```python
from build123d import *

# Parameters (mm, degrees)
EXTRUDE_1_DEPTH     = 2.5
FILLET_1_R          = 5
FILLET_2_R          = 10
FILLET_3_R          = 5
FILLET_4_R          = 1
EXTRUDE_2_DEPTH     = 12
SKETCH_3_R          = 2
CUT_EXTRUDE_1_DEPTH = 128.145329142
SHELL_1_T           = -1.2
CUT_EXTRUDE_2_DEPTH = 127.419500089
SKETCH_5_W          = 29.908945793
SKETCH_5_H          = 26
CUT_EXTRUDE_3_DEPTH = 12
CUT_EXTRUDE_4_DEPTH = 25
SKETCH_7_W          = 24.826968957
SKETCH_7_H          = 53.255380941
CUT_EXTRUDE_5_DEPTH = 140


with BuildPart() as part:
    # 草图1 → 凸台-拉伸1 (new body)
    with BuildSketch(Plane.XY):
        with BuildLine():
            Line((17, 0), (17, 14))
            Line((17, 14), (0, 14))
            Line((0, 14), (0, 43))
            Line((0, 43), (50, 43))
            Line((50, 43), (55, 46))
            Line((55, 46), (117, 46))
            Line((117, 46), (117, 43))
            Line((117, 43), (117, 0))
            ThreePointArc((117, 0), (93.5, -2.800462964), (70, 0))
            Line((70, 0), (17, 0))
        make_face()
    extrude(amount=EXTRUDE_1_DEPTH)

    # 圆角1
    fillet_1_edges = [part.edges().sort_by_distance(p)[0] for p in [
        (17, 0, 1.25),
        (0, 14, 1.25),
        (0, 43, 1.25),
        (117, 46, 1.25),
    ]]
    fillet(fillet_1_edges, radius=FILLET_1_R)

    # 圆角2
    fillet_2_edges = [part.edges().sort_by_distance(p)[0] for p in [
        (117, 0, 1.25),
    ]]
    fillet(fillet_2_edges, radius=FILLET_2_R)

    # 圆角3
    fillet_3_edges = [part.edges().sort_by_distance(p)[0] for p in [
        (70, 0, 1.25),
        (50, 43, 1.25),
        (55, 46, 1.25),
    ]]
    fillet(fillet_3_edges, radius=FILLET_3_R)

    # 圆角4
    fillet_4_edges = [part.edges().sort_by_distance(p)[0] for p in [
        (17, 14, 1.25),
    ]]
    fillet(fillet_4_edges, radius=FILLET_4_R)

    # 草图2 → 凸台-拉伸2 (add)
    with BuildSketch(Plane(origin=(0, 0, 0), x_dir=(-1, 0, 0), z_dir=(0, 0, -1))):
        with BuildLine():
            Line((-51.44480683, 43.283788909), (-54.069688925, 44.858718166))
            ThreePointArc((-54.069688925, 44.858718166), (-55.183718706, 45.336717177), (-56.384919825, 45.5))
            Line((-56.384919825, 45.5), (-112, 45.5))
            ThreePointArc((-112, 45.5), (-115.181980515, 44.181980515), (-116.5, 41))
            Line((-116.5, 41), (-116.5, 8.217797336))
            ThreePointArc((-116.5, 8.217797336), (-114.203731672, 2.024555051), (-108.425, -1.174719632))
            ThreePointArc((-108.425, -1.174719632), (-89.475956652, -2.219058182), (-70.673302226, 0.353309083))
            ThreePointArc((-70.673302226, 0.353309083), (-70.04666276, 0.463204186), (-69.411524962, 0.5))
            Line((-69.411524962, 0.5), (-22, 0.5))
            ThreePointArc((-22, 0.5), (-18.818019485, 1.818019485), (-17.5, 5))
            Line((-17.5, 5), (-17.5, 13))
            ThreePointArc((-17.5, 13), (-17.060660172, 14.060660172), (-16, 14.5))
            Line((-16, 14.5), (-5, 14.5))
            ThreePointArc((-5, 14.5), (-1.818019485, 15.818019485), (-0.5, 19))
            Line((-0.5, 19), (-0.5, 38))
            ThreePointArc((-0.5, 38), (-1.818019485, 41.181980515), (-5, 42.5))
            Line((-5, 42.5), (-48.615080175, 42.5))
            ThreePointArc((-48.615080175, 42.5), (-50.083214876, 42.699567895), (-51.44480683, 43.283788909))
        make_face()
    extrude(amount=EXTRUDE_2_DEPTH)

    # 草图3 → 切除-拉伸1 (cut, through all)
    with BuildSketch(Plane(origin=(0, 45.5, 0), x_dir=(1, 0, 0), z_dir=(0, 1, 0))):
        with Locations(Location((98, 2.5, 0), (0, 0, 270))):
            Circle(SKETCH_3_R)
    extrude(amount=-CUT_EXTRUDE_1_DEPTH, mode=Mode.SUBTRACT)

    # 抽壳1
    shell_1_openings = [part.faces().sort_by_distance(p)[0] for p in [
        (62.500022263, 22.701927877, -12),
    ]]
    offset(amount=SHELL_1_T, openings=shell_1_openings, kind=Kind.INTERSECTION)

    # 草图4 → 切除-拉伸2 (cut, through all)
    with BuildSketch(Plane(origin=(0, 0, 1.3), x_dir=(-1, 0, 0), z_dir=(0, 0, -1))):
        with BuildLine():
            Line((-56.384919825, 44.8), (-112, 44.8))
            ThreePointArc((-112, 44.8), (-114.687005769, 43.687005769), (-115.8, 41))
            Line((-115.8, 41), (-115.8, 8.217797336))
            ThreePointArc((-115.8, 8.217797336), (-113.672930391, 2.48089922), (-108.32, -0.482639434))
            ThreePointArc((-108.32, -0.482639434), (-89.504266505, -1.519630879), (-70.83389206, 1.03463933))
            ThreePointArc((-70.83389206, 1.03463933), (-70.12749848, 1.158521082), (-69.411524962, 1.2))
            Line((-69.411524962, 1.2), (-22, 1.2))
            ThreePointArc((-22, 1.2), (-19.312994231, 2.312994231), (-18.2, 5))
            Line((-18.2, 5), (-18.2, 13))
            ThreePointArc((-18.2, 13), (-17.555634919, 14.555634919), (-16, 15.2))
            Line((-16, 15.2), (-5, 15.2))
            ThreePointArc((-5, 15.2), (-2.312994231, 16.312994231), (-1.2, 19))
            Line((-1.2, 19), (-1.2, 38))
            ThreePointArc((-1.2, 38), (-2.312994231, 40.687005769), (-5, 41.8))
            Line((-5, 41.8), (-48.615080175, 41.8))
            ThreePointArc((-48.615080175, 41.8), (-50.270068383, 42.024967445), (-51.804953859, 42.683543861))
            Line((-51.804953859, 42.683543861), (-54.429835954, 44.258473118))
            ThreePointArc((-54.429835954, 44.258473118), (-55.370572214, 44.662116727), (-56.384919825, 44.8))
        make_face()
    extrude(amount=-CUT_EXTRUDE_2_DEPTH, mode=Mode.SUBTRACT)

    # 草图5 → 切除-拉伸3 (cut)
    with BuildSketch(Plane.XY.offset(2.5)):
        with Locations((94.149762403, 21.5)):
            Rectangle(SKETCH_5_W, SKETCH_5_H)
    extrude(amount=-CUT_EXTRUDE_3_DEPTH, mode=Mode.SUBTRACT)

    # 草图6 → 切除-拉伸4 (cut)
    with BuildSketch(Plane(origin=(0, 46, 0), x_dir=(1, 0, 0), z_dir=(0, 1, 0))):
        with BuildLine():
            add(Edge.make_bspline(
                [(96.996390033, -4.054230802), (96.985471859, -2.387863189), (93.231055265, 1.445134708), (88.130068901, 3.304325139), (82.90634874, 4.073922209), (79.327396591, 1.560107395), (76.925149921, -0.689014198), (71.094345742, -10.024640193), (97.032245655, -9.526634001), (96.996390033, -4.054230802)],
                knots=[0, 0, 0, 0, 0.1331942, 0.239246022, 0.354041302, 0.427365379, 0.493243552, 0.562586095, 1, 1, 1, 1], degree=3))
        make_face()
    extrude(amount=-CUT_EXTRUDE_4_DEPTH, mode=Mode.SUBTRACT)

    # 镜向1: part across plane


with BuildPart() as part_1:
    add(part.part)
    add(part.part.mirror(Plane(origin=(0, 14, 2.5), x_dir=(0, 0, 1), z_dir=(1, 0, 0))))

    # 草图7 → 切除-拉伸5 (cut)
    with BuildSketch(Plane.ZY):
        with Locations((-5.12662644, 20.756877597)):
            Rectangle(SKETCH_7_W, SKETCH_7_H)
    extrude(amount=-CUT_EXTRUDE_5_DEPTH, mode=Mode.SUBTRACT)


solid = part_1.part
```
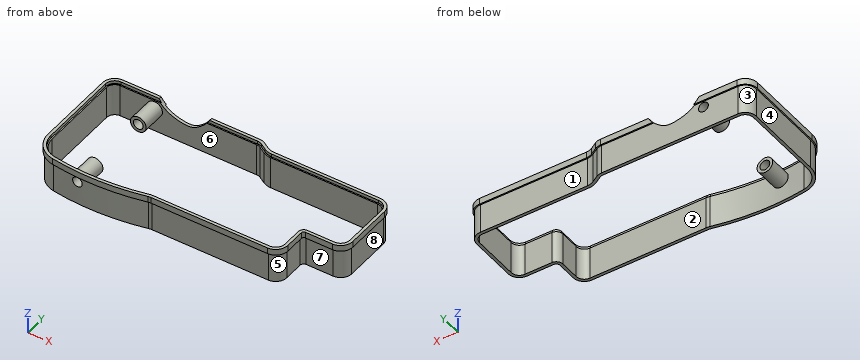
Check sheet for the modelled part. Datum: model origin and axes. Units: mm. Face numbers are marked on the shaded views. A direction names the side the tool comes from. Round coordinates to 2 decimals unless told otherwise and drop trailing zeros. Order: outer loops, then holes, each group sorted by start corner. A loop starts at its lowest first (then second) coordinate and runs counter-clockwise, first axis right, second up. Notation, with made-up numbers: (40, 66.5) - (54, 66.5) arc R28 ccw to (54, 89.5) - close; hole circle Ø7 at (60.25, -26.75). An arc over 180 degrees is marked (long way). Answer as CSV lines item,"result". Start each with the question number.
1) Draft check along X on the marked faces 6, 7 and 8. Enter one of: +X half, -X half, draft (parallel to the pull), parting line (faces both ways), or undercut.
2) Depth check by flat-ended pin: pin 1 (5.5 mm diameter, centred on x = -9, z = -3, fed in from +Y); pin 2 (3.5 mm diameter, centred on x = -8, z = -8.5, fed in from -Y); pin 3 (3 mm diameter, centred on x = -99.5, z = -3, fed in from +Y). Enter the tip coordinate at first touch or a pass-through.
3) Section check A-A (x = -60). Record the cut outline in (y, z).
4) Section check D-D (x = -98). Give the number of separate pieces and of enclosed holes in the cut face, then the cut area to 3 significant figures.
5) Section check B-B (y = 27). Record the cut outline in (x, z), then the cut area to 3 significant figures.
6) Section check C-C (y = 3). Record the cut outline in (x, z), then the cut area to 3 significant figures.
7) Tool access check on the marked faces 1, 2, 3, 4 and 5. Record the directions out of +Z, -Z, +X, -X, +Y, -Y that give a thin tool (end or side, any length) a straight path to the whole face; none if there is none.
8) Scan lines: probe 1 along Z at (x, y) = (-98, 38); probe 2 along Y at (x, z) = (-63, -2.5); probe 3 along Y at (x, z) = (-28.5, -7.5). Record each from-to range of solid material in increasing order.
Determined:
1,face 6,"undercut"
1,face 7,"draft"
1,face 8,"+X half"
2,pin 1,"y = 42.5"
2,pin 2,"y = 14.5"
2,pin 3,"y = 45.5"
3,outline,"(0, 0) - (0.5, 0) - (0.5, -12) - (1.7, -12) - (1.7, 1.2) - (1.2, 1.2) - (1.2, 2.5) - (0, 2.5) - close; (44.3, -12) - (45.5, -12) - (45.5, 0) - (46, 0) - (46, 2.5) - (44.8, 2.5) - (44.8, 1.2) - (44.3, 1.2) - close"
4,separate pieces,"4"
4,enclosed holes,"0"
4,area,"72.7 mm^2"
5,outline,"(-117, 0) - (-116.5, 0) - (-116.5, -12) - (-115.3, -12) - (-115.3, 1.2) - (-115.8, 1.2) - (-115.8, 2.5) - (-117, 2.5) - close; (-1.7, -12) - (-0.5, -12) - (-0.5, 0) - (0, 0) - (0, 2.5) - (-1.2, 2.5) - (-1.2, 1.2) - (-1.7, 1.2) - close"
5,area,"36.0 mm^2"
6,outline,"(-115.53, 0) - (-114.94, 0) - (-114.94, -12) - (-113.45, -12) - (-113.45, 1.2) - (-114.09, 1.2) - (-114.09, 2.5) - (-115.53, 2.5) - close; circle Ø6.4 at (-98, -2.5); (-19.38, -12) - (-17.97, -12) - (-17.97, 0) - (-17.42, 0) - (-17.42, 2.5) - (-18.77, 2.5) - (-18.77, 1.2) - (-19.38, 1.2) - close; hole circle Ø4 at (-98, -2.5)"
6,area,"62.8 mm^2"
7,face 1,"-Z, +X, +Y"
7,face 2,"+Z, -Z"
7,face 3,"-Z, -X, +Y"
7,face 4,"-Z, -X, +Y, -Y"
7,face 5,"-Z, +X, -Y"
8,probe 1,"-5.7 to -4.5, -0.5 to 0.7"
8,probe 2,"0.5 to 1.7, 44.3 to 45.5"
8,probe 3,"0.5 to 1.7, 41.3 to 42.5"
